Part model, mm, in its own coordinate system. Round coordinates to 2 decimals unless told otherwise and drop trailing zeros. Loops run counter-clockwise (first coordinate to the right, second up) from the corner with the lowest first, then second, coordinate; pieces in that order, holes last.
from build123d import *

# Parameters (mm, degrees)
SKETCH1_W           = 225
SKETCH1_H           = 65
SKETCH1_R           = 3.75
SKETCH1_R_2         = 5.177315147
SKETCH1_R_3         = 5.175
SKETCH1_R_4         = 3.445800431
BOSS_EXTRUDE1_DEPTH = 6
CHAMFER1_SIZE       = 10
CUT_EXTRUDE1_REACH  = 119.742
SKETCH3_R           = 1.55
SKETCH3_R_2         = 11.5


with BuildPart() as part:
    # Sketch1 → Boss-Extrude1 (new body)
    with BuildSketch(Plane.XY):
        with Locations((0, 1.720251483)):
            Rectangle(SKETCH1_W, SKETCH1_H)
        with Locations((83.5, -20.779748517)):
            Circle(SKETCH1_R, mode=Mode.SUBTRACT)
        with Locations((51.5, -20.779748517)):
            Circle(SKETCH1_R, mode=Mode.SUBTRACT)
        with Locations((67.5, -20.779748517)):
            Circle(SKETCH1_R_2, mode=Mode.SUBTRACT)
        with Locations((-51.5, -20.779748517)):
            Circle(SKETCH1_R, mode=Mode.SUBTRACT)
        with Locations((-83.5, -20.779748517)):
            Circle(SKETCH1_R, mode=Mode.SUBTRACT)
        with Locations((-67.5, -20.779748517)):
            Circle(SKETCH1_R_3, mode=Mode.SUBTRACT)
        with Locations((30, -20.779748517)):
            Circle(SKETCH1_R_4, mode=Mode.SUBTRACT)
        with Locations((-30, -20.779748517)):
            Circle(SKETCH1_R_4, mode=Mode.SUBTRACT)
        with Locations((100, -20.779748517)):
            Circle(SKETCH1_R_4, mode=Mode.SUBTRACT)
        with Locations((100, 24.220251483)):
            Circle(SKETCH1_R_4, mode=Mode.SUBTRACT)
        with Locations((-0.222785291, 24.220251483)):
            Circle(SKETCH1_R_4, mode=Mode.SUBTRACT)
        with Locations((-100, -20.779748517)):
            Circle(SKETCH1_R_4, mode=Mode.SUBTRACT)
        with Locations((-100, 24.220251483)):
            Circle(SKETCH1_R_4, mode=Mode.SUBTRACT)
    extrude(amount=BOSS_EXTRUDE1_DEPTH)

    # Chamfer1
    chamfer1_edges = [part.edges().sort_by_distance(p)[0] for p in [
        (112.5, 34.220251483, 3),
        (112.5, -30.779748517, 3),
        (-112.5, -30.779748517, 3),
        (-112.5, 34.220251483, 3),
    ]]
    chamfer(chamfer1_edges, length=CHAMFER1_SIZE)

    # Sketch3 → Cut-Extrude1 (cut, up to next)
    with BuildSketch(Plane.XY.offset(6), mode=Mode.PRIVATE) as cut_extrude1_sk1:
        with Locations((-15.680841051, -25.279748517)):
            Circle(SKETCH3_R)
    cut_extrude1_tool1 = extrude(cut_extrude1_sk1.sketch, amount=-CUT_EXTRUDE1_REACH, mode=Mode.PRIVATE) & part.part
    # Sketch3 → Cut-Extrude1 (cut, up to next)
    with BuildSketch(Plane.XY.offset(6), mode=Mode.PRIVATE) as cut_extrude1_sk2:
        with Locations((-15.680841051, 5.720251483)):
            Circle(SKETCH3_R)
    cut_extrude1_tool2 = extrude(cut_extrude1_sk2.sketch, amount=-CUT_EXTRUDE1_REACH, mode=Mode.PRIVATE) & part.part
    # Sketch3 → Cut-Extrude1 (cut, up to next)
    with BuildSketch(Plane.XY.offset(6), mode=Mode.PRIVATE) as cut_extrude1_sk3:
        with Locations((15.319158949, 5.720251483)):
            Circle(SKETCH3_R)
    cut_extrude1_tool3 = extrude(cut_extrude1_sk3.sketch, amount=-CUT_EXTRUDE1_REACH, mode=Mode.PRIVATE) & part.part
    # Sketch3 → Cut-Extrude1 (cut, up to next)
    with BuildSketch(Plane.XY.offset(6), mode=Mode.PRIVATE) as cut_extrude1_sk4:
        with Locations((15.319158949, -25.279748517)):
            Circle(SKETCH3_R)
    cut_extrude1_tool4 = extrude(cut_extrude1_sk4.sketch, amount=-CUT_EXTRUDE1_REACH, mode=Mode.PRIVATE) & part.part
    # Sketch3 → Cut-Extrude1 (cut, up to next)
    with BuildSketch(Plane.XY.offset(6), mode=Mode.PRIVATE) as cut_extrude1_sk5:
        with Locations((-0.180841051, -9.779748517)):
            Circle(SKETCH3_R_2)
    cut_extrude1_tool5 = extrude(cut_extrude1_sk5.sketch, amount=-CUT_EXTRUDE1_REACH, mode=Mode.PRIVATE) & part.part
    add(cut_extrude1_tool1.solids().sort_by_distance((-15.680841, -25.279749, 6))[0], mode=Mode.SUBTRACT)
    add(cut_extrude1_tool2.solids().sort_by_distance((-15.680841, 5.720251, 6))[0], mode=Mode.SUBTRACT)
    add(cut_extrude1_tool3.solids().sort_by_distance((15.319159, 5.720251, 6))[0], mode=Mode.SUBTRACT)
    add(cut_extrude1_tool4.solids().sort_by_distance((15.319159, -25.279749, 6))[0], mode=Mode.SUBTRACT)
    add(cut_extrude1_tool5.solids().sort_by_distance((-0.180841, -9.779749, 6))[0], mode=Mode.SUBTRACT)


solid = part.part
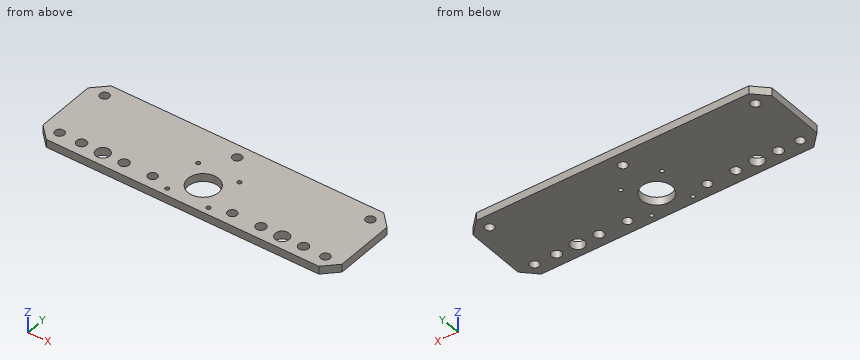
1) Wall check: line 1 along X through (y, z) = (24, 2); line 2 along Y through (x, z) = (-50, 0.7); line 3 along X through (y, z) = (23, 5.15). Give the ranges that are in metal, low to high.
Values:
line 1: x = -112.5 to -103.44, -96.56 to -3.66, 3.22 to 96.56, 103.44 to 112.5
line 2: y = -30.78 to -24.22, -17.34 to 34.22
line 3: x = -112.5 to -103.22, -96.78 to -3.45, 3 to 96.78, 103.22 to 112.5
2) Slice it at A-A, the plane x = 83.5. Give the cut face in (y, z), then the cut area to 3 significant figures.
Values:
outline: (-30.78, 0) - (-24.53, 0) - (-24.53, 6) - (-30.78, 6) - close; (-17.03, 0) - (34.22, 0) - (34.22, 6) - (-17.03, 6) - close
area: 345 mm2
3) Slice it at D-D, the plane y = 30. Give the cut face in (x, z), then the cut area to 3 significant figures.
Values:
outline: (-106.72, 0) - (106.72, 0) - (106.72, 6) - (-106.72, 6) - close
area: 1,280 mm2
4) Slice it at B-B, the plane x = -67.5. Give the cut face in (y, z), then the cut area to 3 significant figures.
Values:
outline: (-30.78, 0) - (-25.95, 0) - (-25.95, 6) - (-30.78, 6) - close; (-15.6, 0) - (34.22, 0) - (34.22, 6) - (-15.6, 6) - close
area: 328 mm2
5) Slice it at C-C, the plane z = 1.05. Give the number of separate pieces and of enclosed holes in the cut face, then the cut area to 3 significant figures.
Values:
separate pieces: 1
enclosed holes: 18
area: 13,400 mm2
